Geometry: final body of the model. Coordinates: model frame, mm. A direction names the side the tool comes from. Coordinates: 2 decimals unless noted, no trailing zeros. Write each loop counter-clockwise with the first axis right and the second up, starting at its lowest first coordinate (ties: lowest second). Pieces come first, ordered by that corner, then holes. Notation, with made-up numbers: (56.25, -3.75) - (80.25, -3.75) arc R8 ccw to (80.25, 3.25) - close; hole circle Ø5 at (-32.5, 26). An arc over 180 degrees is marked (long way). Answer as a JSON object with one key per item and string values. Group by question number.
Item 1: Section B-B on x = 0. Return loops of the section in (y, z), and give its area (3 significant figures).
Item 2: Set-up query: faces 5 (the flat face through (-90, 10, -50)), 6 (the flat face through (90, 10, 50)), 7 (the flat face through (60, 10, -62)), 8 (the flat face through (60, 10, 63)), 9 (the flat face through (-80, 10, 63)). Return all of +Z, -Z, +X, -X, +Y, -Y with unobstructed straight access to the full face (end or side cutting, diameter ignored); none if empty.
Item 3: Section C-C on y = 5.75. Return loops of the section in (x, z), and give its area (3 significant figures).
Item 4: First-contact query: pin 1 Ø6 at (x, y) = (94.5, 7.5) entering from -Z; pin 2 Ø10 at (x, y) = (41.5, 4) entering from +Z; pin 3 Ø10 at (y, z) = (8, -62.5) entering from +X; pin 4 Ø12 at (y, z) = (8.5, 27) entering from -X. Flat tips, straight axial feed; report the tip coordinate or a pass-through.
Item 5: Mould query, pull axis X, two halves, no side actions, for faces 1 (the flat face through (-1, 20, -16)), 2 (the flat face through (-80, 10, -62)), 3 (the flat face through (-1, 10, -50)), 4 (the cylindrical face through (96.99, 2.85, -0.7)). Classes: pulls with the +X half, pulls with the -X half, needs draft (parallel to the pull), parting line crosses it, or undercut.
Item 6: Line query: line 1 along X through (y, z) = (19, 61.5); line 2 along X through (y, z) = (4, -64); line 3 along X through (y, z) = (17, -54). Output: solid intervals per line, ascending. Write a range as from..to.
Item 7: Section D-D on y = 25.5. Return loops of the section in (x, z).
```python
from build123d import *

# Parameters (mm, degrees)
SKETCH1_W           = 200
SKETCH1_H           = 100
BOSS_EXTRUDE1_DEPTH = 20
SKETCH2_W           = 20
SKETCH2_H           = 20
BOSS_EXTRUDE2_DEPTH = 75
SKETCH3_W           = 20
SKETCH3_H           = 20
BOSS_EXTRUDE3_DEPTH = 75
SKETCH4_R           = 8
CUT_EXTRUDE1_DEPTH  = 150
SKETCH5_R           = 5
BOSS_EXTRUDE4_DEPTH = 30
FILLET3_R           = 10
FILLET4_R           = 10


with BuildPart() as part:
    # Sketch1 → Boss-Extrude1 (new body)
    with BuildSketch(Plane(origin=(0, 0, 0), x_dir=(1, 0, 0), z_dir=(0, 1, 0))):
        Rectangle(SKETCH1_W, SKETCH1_H)
    extrude(amount=BOSS_EXTRUDE1_DEPTH)

    # Sketch2 → Boss-Extrude2 (add, symmetric)
    with BuildSketch(Plane.XY):
        with Locations((-70, 10)):
            Rectangle(SKETCH2_W, SKETCH2_H)
    extrude(amount=BOSS_EXTRUDE2_DEPTH, both=True)

    # Sketch3 → Boss-Extrude3 (add, symmetric)
    with BuildSketch(Plane.XY):
        with Locations((70, 10)):
            Rectangle(SKETCH3_W, SKETCH3_H)
    extrude(amount=BOSS_EXTRUDE3_DEPTH, both=True)

    # Sketch4 → Cut-Extrude1 (cut)
    with BuildSketch(Plane(origin=(0, 0, 0), x_dir=(1, 0, 0), z_dir=(0, 1, 0))):
        with Locations(Location((-70.221727327, 65.616664793, 0), (0, 0, 270))):
            Circle(SKETCH4_R)
        with Locations(Location((70.221727327, 65.616664793, 0), (0, 0, 270))):
            Circle(SKETCH4_R)
        with Locations(Location((-70.221727327, -65.616664793, 0), (0, 0, 270))):
            Circle(SKETCH4_R)
        with Locations(Location((70.221727327, -65.616664793, 0), (0, 0, 270))):
            Circle(SKETCH4_R)
    extrude(amount=CUT_EXTRUDE1_DEPTH, mode=Mode.SUBTRACT)

    # Sketch5 → Boss-Extrude4 (add)
    with BuildSketch(Plane(origin=(0, 0, 0), x_dir=(1, 0, 0), z_dir=(0, 1, 0))):
        with Locations(Location((0, 0, 0), (0, 0, 270))):
            Circle(SKETCH5_R)
    extrude(amount=BOSS_EXTRUDE4_DEPTH)

    # Fillet3
    fillet3_edges = [part.edges().sort_by_distance(p)[0] for p in [
        (100, 0, 0),
        (100, 20, 0),
    ]]
    fillet(fillet3_edges, radius=FILLET3_R - 0.0001)  # a hair under: the kernel refuses the full size

    # Fillet4
    fillet4_edges = [part.edges().sort_by_distance(p)[0] for p in [
        (-100, 0, 0),
        (-100, 20, 0),
    ]]
    fillet(fillet4_edges, radius=FILLET4_R - 0.0001)  # a hair under: the kernel refuses the full size


solid = part.part
```
Checks:
{
 "1": {"outline": "(0, -50) - (20, -50) - (20, -5) - (30, -5) - (30, 5) - (20, 5) - (20, 50) - (0, 50) - close", "area": "2,100 mm^2"},
 "2": {"face 5": "-Z, -X, +Y, -Y", "face 6": "+Z, +X, +Y, -Y", "face 7": "-Z, +Y, -Y", "face 8": "+Z, +Y, -Y", "face 9": "+Z, -X, +Y, -Y"},
 "3": {"outline": "(-99.05, -50) - (-80, -50) - (-80, -75) - (-60, -75) - (-60, -50) - (60, -50) - (60, -75) - (80, -75) - (80, -50) - (99.05, -50) - (99.05, 50) - (80, 50) - (80, 75) - (60, 75) - (60, 50) - (-60, 50) - (-60, 75) - (-80, 75) - (-80, 50) - (-99.05, 50) - close; hole circle Ø16 at (-70.22, -65.62); hole circle Ø16 at (-70.22, 65.62); hole circle Ø16 at (70.22, -65.62); hole circle Ø16 at (70.22, 65.62)", "area": "21,000 mm^2"},
 "4": {"pin 1": "z = -50", "pin 2": "z = 50", "pin 3": "x = 80", "pin 4": "x = -100"},
 "5": {"face 1": "needs draft", "face 2": "pulls with the -X half", "face 3": "undercut", "face 4": "pulls with the +X half"},
 "6": {"line 1": "-80..-77.08, -63.36..-60, 60..63.36, 77.08..80", "line 2": "-80..-78.06, -62.39..-60, 60..62.39, 78.06..80", "line 3": "-80..-60, 60..80"},
 "7": {"outline": "circle Ø10 at (0, 0)"}
}
